For this review, take the finished solid that the model builds, in its own axes (mm). Face numbers are marked on the shaded views. Round coordinates to 2 decimals unless told otherwise and drop trailing zeros. Loops run counter-clockwise (first coordinate to the right, second up) from the corner with the lowest first, then second, coordinate; pieces in that order, holes last. Notation, with made-up numbers: (28, 26) -> (69, 26) arc R21 ccw to (69, 31) -> close; hole circle Ø5 at (67.5, 67.25). An arc over 180 degrees is marked (long way). Write each question's results on one line, items separated by ' | '.
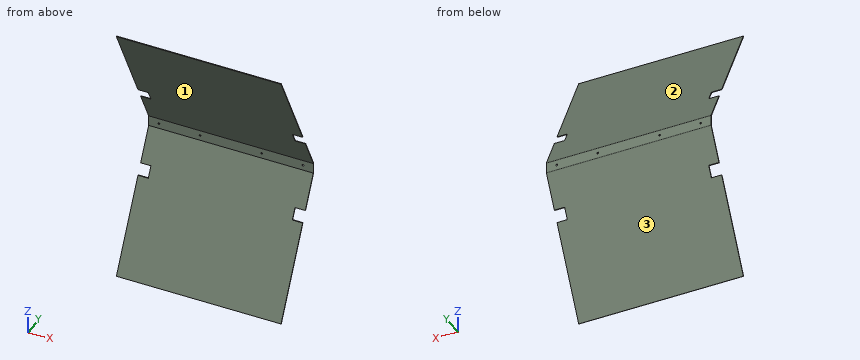
Autodesk Inventor part; units mm, degrees
ref_plane "YZ Plane" through (0, 0, 0) normal (1, 0, 0) x (0, 1, 0)
ref_plane "XZ Plane" through (0, 0, 0) normal (0, 1, 0) x (-1, 0, 0)
ref_plane "XY Plane" through (0, 0, 0) normal (0, 0, 1) x (1, 0, 0)
sketch "Sketch1" plane through (0, 0, 0) normal (0, 1, 0) x (-1, 0, 0)
  line L0 (203.2, 12.7) -> (-203.2, 12.7)
  line L1 (-203.2, 12.7) -> (-203.2, -12.7)
  line L2 (-203.2, -12.7) -> (203.2, -12.7)
  line L3 (203.2, -12.7) -> (203.2, 12.7)
  line L4 (203.2, 12.7) -> (-203.2, -12.7) construction
  line L5 (-203.2, 12.7) -> (203.2, -12.7) construction
  point P0 (0, 0)
  dimension "d0" = 406.4
  dimension "d1" = 25.4
extrude "Extrusion1" add sketch "Sketch1" along normal blind 1.5875
sketch "Sketch2" plane through (0, 1.5875, 0) normal (0, 1, 0) x (1, 0, 0)
  line L0 (-203.2, 12.7) -> (-203.2, -12.7)
  line L1 (203.2, -12.7) -> (203.2, 12.7)
  point P0 (0, 0)
  point P1 (-177.8, 0)
  point P2 (-152.4, 0)
  point P3 (177.8, 0)
  point P4 (152.4, 0)
  point P5 (76.2, 0)
  point P6 (50.8, 0)
  point P7 (-76.2, 0)
  point P8 (-50.8, 0)
  dimension "d4" = 25.4
  dimension "d5" = 25.4
  dimension "d6" = 25.4
  dimension "d7" = 25.4
  dimension "d8" = 25.4
  dimension "d9" = 25.4
  dimension "d10" = 76.2
  dimension "d11" = 76.2
hole "Hole1" at (-177.8, 1.5875, 0) at (177.8, 1.5875, 0) at (76.2, 1.5875, 0) at (-76.2, 1.5875, 0) direction (0, -1, 0) diameter 4.318 end through all
sketch "Sketch3" plane through (203.2, 0, 12.7) normal (1, 0, 0) x (0, 0, -1)
  line L0 (0, 0) -> (25.4, 0)
  line L1 (0, 0) -> (-0.7189, 1.4154)
  line L2 (-0.7189, 1.4154) -> (-307.7868, -154.5406)
  line L3 (-307.7868, -154.5406) -> (-307.068, -155.956)
  line L4 (-307.068, -155.956) -> (0, 0)
  line L5 (25.4, 0) -> (26.1189, 1.4154)
  line L6 (26.1189, 1.4154) -> (333.1868, -154.5406)
  line L7 (333.1868, -154.5406) -> (332.468, -155.956)
  line L8 (332.468, -155.956) -> (25.4, 0)
  line L9 (0, 0) -> (0, 1.5875)
  line L10 (25.4, 0) -> (25.4, 1.5875)
  line L11 (0, 1.5875) -> (25.4, 1.5875)
  arc A0 (0, 1.5875) -> (-0.7189, 1.4154) centre (0, 0) ccw
  arc A1 (26.1189, 1.4154) -> (25.4, 1.5875) centre (25.4, 0) ccw
  line L12 (-204.5453, -103.886) -> (-179.1453, -103.886)
  line L13 (-357.0791, -181.356) -> (382.4791, -181.356)
  point P0 (12.7, 0)
  point P1 (12.7, -181.356)
  point P2 (12.7, 0)
  dimension "d19" = 25.4
  dimension "d20" = 103.886
  dimension "d21" = 207.0877
  dimension "d22" = 181.356
  dimension "d23" = 25.4
extrude "Extrusion2" add sketch "Sketch3" against normal up to surface (406.4 mm away) contours L4 L3 L2 L1 | L1 A0 L9 | L10 A1 L5 | L5 L6 L7 L8
sketch "Sketch4" plane through (0, 1.5875, 0) normal (0, 1, 0) x (1, 0, 0)
  line L0 (203.2, -319.768) -> (203.2, -12.7)
  line L1 (203.2, -88.9) -> (177.8, -88.9)
  line L2 (177.8, -88.9) -> (177.8, -114.3)
  line L3 (177.8, -114.3) -> (203.2, -114.3)
  line L4 (203.2, -114.3) -> (203.2, -88.9)
  line L5 (203.2, 12.7) -> (203.2, 319.768)
  line L6 (203.2, 88.9) -> (177.8, 88.9)
  line L7 (177.8, 88.9) -> (177.8, 114.3)
  line L8 (177.8, 114.3) -> (203.2, 114.3)
  line L9 (203.2, 114.3) -> (203.2, 88.9)
  line L10 (-203.2, 12.7) -> (-203.2, 319.768)
  line L11 (-203.2, 114.3) -> (-177.8, 114.3)
  line L12 (-177.8, 114.3) -> (-177.8, 88.9)
  line L13 (-177.8, 88.9) -> (-203.2, 88.9)
  line L14 (-203.2, 88.9) -> (-203.2, 114.3)
  line L15 (-203.2, -319.768) -> (-203.2, -12.7)
  line L16 (-203.2, -88.9) -> (-177.8, -88.9)
  line L17 (-177.8, -88.9) -> (-177.8, -114.3)
  line L18 (-177.8, -114.3) -> (-203.2, -114.3)
  line L19 (-203.2, -114.3) -> (-203.2, -88.9)
  line L20 (177.8, -88.9) -> (177.8, 88.9) construction
  line L21 (-177.8, 88.9) -> (-177.8, -88.9) construction
  point P0 (0, 0)
  point P1 (-177.8, 0)
  point P2 (177.8, 0)
  point P3 (177.8, -101.6)
  dimension "d26" = 25.4
  dimension "d29" = 101.6
extrude "Extrusion3" cut sketch "Sketch4" against normal through all
properties part number "Ramp Using 1__16 Gray Tinted Polycarbonate Sheet (36 x 72) (217-6627)" material "Polycarbonate, Clear"
1. Consider section B-B (x = 141). State the section outline as (y, z) points.
Values found:
outline: (-155.96, -319.77) -> (-154.54, -320.49) -> (1.42, -13.42) arc R1.59 ccw to (1.59, -12.7) -> (1.59, 12.7) arc R1.59 ccw to (1.42, 13.42) -> (-154.54, 320.49) -> (-155.96, 319.77) -> (0, 12.7) -> (0, -12.7) -> close
2. To check wall thickness, follow probe 1 along X at (y, z) = (1, 0); probe 2 along Z at (x, y) = (77.5, -122); probe 3 along Z at (x, y) = (76.2, 0.8). State the ranges of each line that lie inside material, in increasing order.
Values found:
probe 1: x = -203.2 to -179.96, -175.64 to -78.36, -74.04 to 74.04, 78.36 to 175.64, 179.96 to 203.2 | probe 2: z = -256.42 to -252.91, 252.91 to 256.42 | probe 3: z = -14.63 to -2.16, 2.16 to 14.63
3. Consider section C-C (y = -62). State the section outline as (x, z) points.
Values found:
outline: (-203.2, -138.28) -> (203.2, -138.28) -> (203.2, -134.77) -> (-203.2, -134.77) -> close; (-203.2, 134.77) -> (203.2, 134.77) -> (203.2, 138.28) -> (-203.2, 138.28) -> close
4. Consider section D-D (z = -241.5). State the section outline as (x, y) points.
Values found:
outline: (-203.2, -116.2) -> (203.2, -116.2) -> (203.2, -114.42) -> (-203.2, -114.42) -> close
5. Consider section A-A (y = -95.5). State the section outline as (x, z) points, plus the area to 3 significant figures.
Values found:
outline: (-203.2, -204.24) -> (203.2, -204.24) -> (203.2, -200.73) -> (-203.2, -200.73) -> close; (-203.2, 200.73) -> (203.2, 200.73) -> (203.2, 204.24) -> (-203.2, 204.24) -> close | area: 2,850 mm2
6. Draft analysis for pull direction Z (two halves, no side actions). For the marked faces 1, 2 and 3, state which applies: released by +Z, released by -Z, zero draft, split by the parting line, or undercut.
Values found:
face 1: undercut | face 2: released by +Z | face 3: released by -Z
7. For pin 1 (1.4 mm diameter, centred on x = 189.5, y = -51, fed in from -Z); pin 2 (11.5 mm diameter, centred on y = -45.5, z = 95.5, fed in from -X); pin 3 (11.5 mm diameter, centred on y = -41, z = 99, fed in from +X), all flat-tipped, find the tip position at first contact; note any pin that passes through.
Values found:
pin 1: stops at z = -118 | pin 2: stops at x = -177.8 | pin 3: stops at x = 177.8
